```python
from build123d import *

# Parameters (mm, degrees)
SKETCH1_W                      = 160
SKETCH1_H                      = 40
BOSS_EXTRUDE1_DEPTH            = 12
M6_CLEARANCE_HOLE1_D           = 7
CBORE_FOR_M4_SHCS1_D           = 4.8
CBORE_FOR_M4_SHCS1_CBORE_D     = 8
CBORE_FOR_M4_SHCS1_CBORE_DEPTH = 4


with BuildPart() as part:
    # Sketch1 → Boss-Extrude1 (new body)
    with BuildSketch(Plane.XY):
        Rectangle(SKETCH1_W, SKETCH1_H)
    extrude(amount=BOSS_EXTRUDE1_DEPTH)

    # M6 Clearance Hole1 (through all)
    with Locations(Plane.XY.offset(12)):
        with Locations((-72.5, 0), (72.5, 0)):
            Hole(M6_CLEARANCE_HOLE1_D / 2)

    # CBORE for M4 SHCS1 (through all)
    with Locations(Plane(origin=(0, 0, 0), x_dir=(-1, 0, 0), z_dir=(0, 0, -1))):
        with Locations((-39.5, 0), (39.5, 0)):
            CounterBoreHole(CBORE_FOR_M4_SHCS1_D / 2, CBORE_FOR_M4_SHCS1_CBORE_D / 2, CBORE_FOR_M4_SHCS1_CBORE_DEPTH)


solid = part.part
```
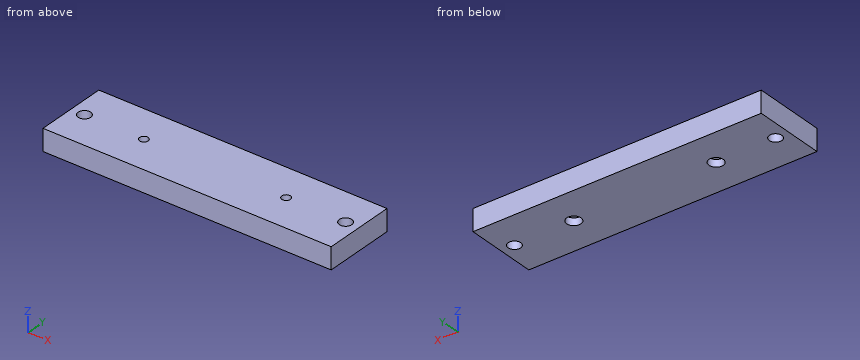
Verification items for the finished model (mm, model axes). Give positions to 0.01 mm unless a question says otherwise; leave off trailing zeros. Order: outer loops, then holes, each group sorted by start corner. A loop starts at its lowest first (then second) coordinate and runs counter-clockwise, first axis right, second up. Notation, with made-up numbers: M 62,-38 L 112,-38 A22 cw 112,-15 Z; hole C 47,9 d9. An arc over 180 degrees is marked long. Answer in a Markdown table with one row per item. Add a question column.
Item 1: Section check A-A, the plane x = -72.5. Enter the section's corners in (y, z), and give its area (3 significant figures).
Item 2: Scan lines: probe 1 along Y at (x, z) = (39.5, 2.9); probe 2 along X at (y, z) = (2.5, 1.75); probe 3 along Y at (x, z) = (-39.5, 9.75). Record each from-to range of solid material in increasing order. Write a range as from..to.
Item 3: Section check D-D, the plane z = 1.5. Enter the section's corners in (x, y).
Item 4: Gauge pin test, flat end, axial feed: pin 1 (6.5 mm diameter, centred on x = -39.5, y = 0, fed in from -Z). Record the tip position at first contact, or that the pin passes through.
Item 5: Section check B-B, the plane z = 10.25. Enter the section's corners in (x, y).
Item 6: Section check C-C, the plane x = 39.5. Enter the section's corners in (y, z), and give its area (3 significant figures).
Filled sheet:
| question | item | result |
|---|---|---|
| 1 | outline | M -20,0 L -3.5,0 L -3.5,12 L -20,12 Z; M 3.5,0 L 20,0 L 20,12 L 3.5,12 Z |
| 1 | area | 396 mm^2 |
| 2 | probe 1 | y = -20..-4, 4..20 |
| 2 | probe 2 | x = -80..-74.95, -70.05..-42.62, -36.38..36.38, 42.62..70.05, 74.95..80 |
| 2 | probe 3 | y = -20..-2.4, 2.4..20 |
| 3 | outline | M -80,-20 L 80,-20 L 80,20 L -80,20 Z; hole C -72.5,0 d7; hole C -39.5,0 d8; hole C 39.5,0 d8; hole C 72.5,0 d7 |
| 4 | pin 1 | stops at z = 4 |
| 5 | outline | M -80,-20 L 80,-20 L 80,20 L -80,20 Z; hole C -72.5,0 d7; hole C -39.5,0 d4.8; hole C 39.5,0 d4.8; hole C 72.5,0 d7 |
| 6 | outline | M -20,0 L -4,0 L -4,4 L -2.4,4 L -2.4,12 L -20,12 Z; M 2.4,4 L 4,4 L 4,0 L 20,0 L 20,12 L 2.4,12 Z |
| 6 | area | 410 mm^2 |
